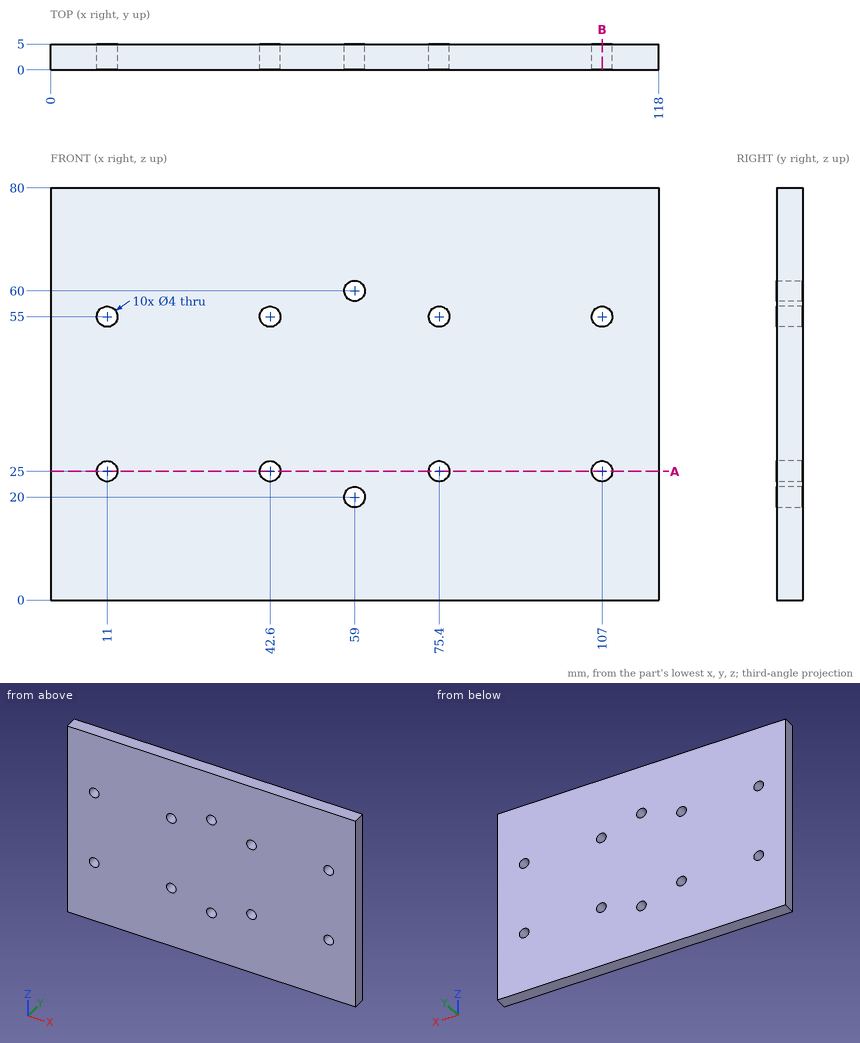
Can you work these out from the drawing? Everything is in mm from the part's minimum corner. Coordinates: 2 decimals unless noted, no trailing zeros. Order: outer loops, then holes, each group sorted by start corner. A loop starts at its lowest first (then second) coordinate and runs counter-clockwise, first axis right, second up. Notation, with made-up numbers: M 40.5,47.5 L 66.5,47.5 A5 cw 66.5,55.5 Z; hole C -27,6 d11. An arc over 180 degrees is marked long. Answer as CSV lines item,"result". Start each with the question number.
1. I need wall thicknesses on line 1 (X direction, y = 3.4, z = 55); line 2 (X direction, y = 1.15, z = 26.5); line 3 (X direction, y = 2.2, z = 20). Which ranges of each line are inside material? Lowest first, please. Write a range as [from, to].
2. I want a section at B-B, the plane x = 107. Write out the boundary of the cut face in (y, z).
3. I want a section at A-A, the plane z = 25. Write out the boundary of the cut face in (x, y).
4. For pin 1 (5 mm diameter, centred on x = 11, z = 25, fed in from -Y), with a flat end and sliding along its axis, tell me the tip position at first contact or that it passes through.
Recorded:
1,line 1,"x = [0, 9], [13, 40.6], [44.6, 73.4], [77.4, 105], [109, 118]"
1,line 2,"x = [0, 9.68], [12.32, 41.28], [43.92, 74.08], [76.72, 105.68], [108.32, 118]"
1,line 3,"x = [0, 57], [61, 118]"
2,outline,"M 0,0 L 5,0 L 5,23 L 0,23 Z; M 0,27 L 5,27 L 5,53 L 0,53 Z; M 0,57 L 5,57 L 5,80 L 0,80 Z"
3,outline,"M 0,0 L 9,0 L 9,5 L 0,5 Z; M 13,0 L 40.6,0 L 40.6,5 L 13,5 Z; M 44.6,0 L 73.4,0 L 73.4,5 L 44.6,5 Z; M 77.4,0 L 105,0 L 105,5 L 77.4,5 Z; M 109,0 L 118,0 L 118,5 L 109,5 Z"
4,pin 1,"stops at y = 0"
